Could you check a few things on this drawing? It's one solid part, dimensions in mm from its lowest x, y, z. A direction names the side the tool comes from. Round coordinates to 2 decimals unless told otherwise and drop trailing zeros. Write each loop counter-clockwise with the first axis right and the second up, starting at its lowest first coordinate (ties: lowest second). Pieces come first, ordered by that corner, then holes. Notation, with made-up numbers: (-27.5, 62) - (28.5, 62) arc R20 ccw to (28.5, 84) - close; hole circle Ø11 at (-6.5, 19.5). An arc over 180 degrees is marked (long way). Write item = value, one per line. Start each with the question number.
Item 1: If we section it at D-D (z = 48): Please give me the cut outline in (x, y), and give its area (3 significant figures).
Item 2: For P1, Ø24, axis at x = 50, z = 32, coming from the +Y side; P2, Ø5, axis at y = 9.5, z = 37.5, coming from the -X side; P3, Ø4, axis at x = 17, y = 3.5, coming from the -Z side; P4, Ø1.5, axis at x = 9.5, y = 8, coming from the +Z side, each with a flat end and sliding along its axis, tell me the tip position at first contact or that it passes through.
Item 3: If we section it at A-A (y = 12): Please give me the cut outline in (x, z).
Item 4: Thinking about a two-plate mould opening in Z: for the marked faces 5, 6 and 7, which applies, pulls with the +Z half, pulls with the -Z half, needs draft (parallel to the pull), parting line crosses it, or undercut?
Item 5: If I drill on line 1 along Z through (x, y) = (68, 18.8); line 2 along Z through (x, y) = (58, 3.05); line 3 along X through (y, z) = (19, 48.5), over which ranges is the centre line in solid material (lowest first)? Write a range as [from, to].
Item 6: Which directions (+Z, -Z, +X, -X, +Y, -Y) give clear straight access to the entire face, cutting with the end or side of a thin tool? Please do the marked faces 1, 2, 3 and 4.
Item 7: If we section it at C-C (z = 16): Please give me the cut outline in (x, y).
Item 8: If we section it at B-B (x = 58): Please give me the cut outline in (y, z), and give its area (3 significant figures).
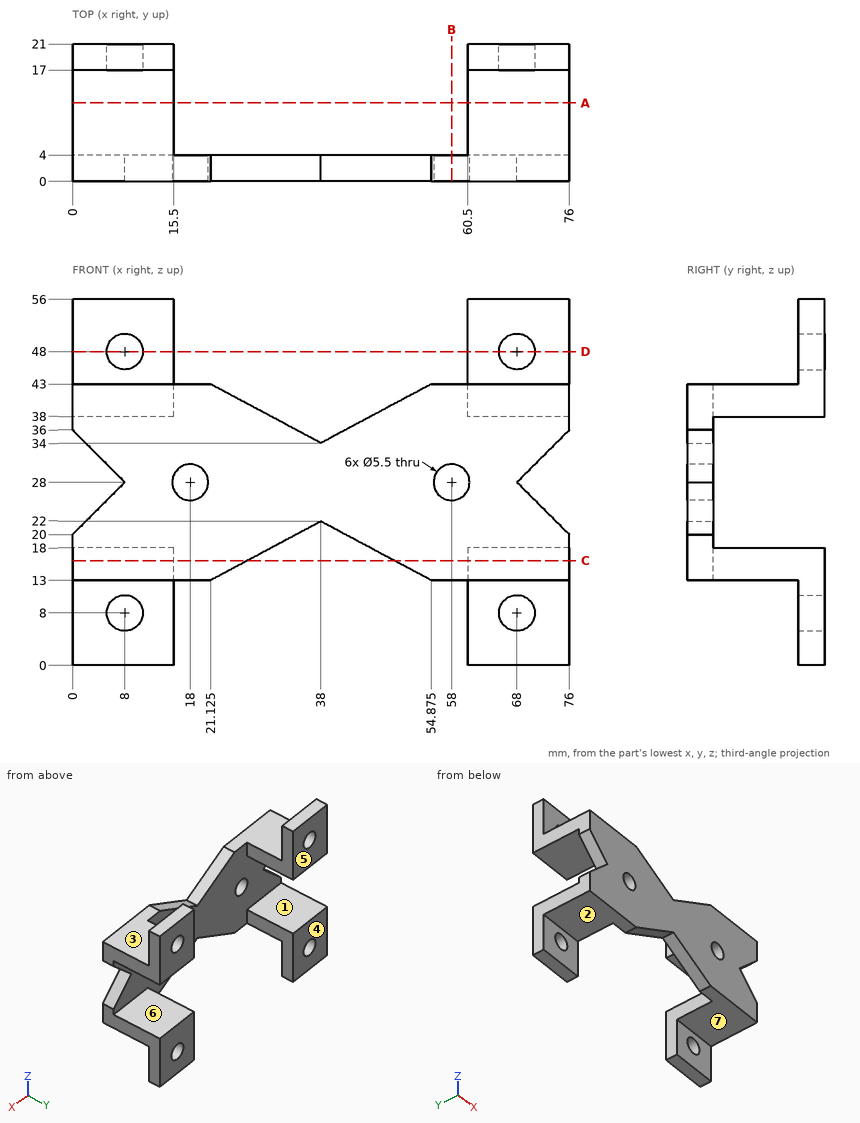
Reply:
q1.outline = (0, 17) - (5.25, 17) - (5.25, 21) - (0, 21) - close; (10.75, 17) - (15.5, 17) - (15.5, 21) - (10.75, 21) - close; (60.5, 17) - (65.25, 17) - (65.25, 21) - (60.5, 21) - close; (70.75, 17) - (76, 17) - (76, 21) - (70.75, 21) - close
q1.area = 80.0 mm2
q2.P1 = 4
q2.P2 = 0
q2.P3 = 13
q2.P4 = 43
q3.outline = (0, 13) - (15.5, 13) - (15.5, 18) - (0, 18) - close; (0, 38) - (15.5, 38) - (15.5, 43) - (0, 43) - close; (60.5, 13) - (76, 13) - (76, 18) - (60.5, 18) - close; (60.5, 38) - (76, 38) - (76, 43) - (60.5, 43) - close
q4.face_5 = needs draft
q4.face_6 = undercut
q4.face_7 = pulls with the -Z half
q5.line_1 = [0, 5.25], [10.75, 18], [38, 45.25], [50.75, 56]
q5.line_2 = [13, 25.25], [30.75, 43]
q5.line_3 = [0, 5.3], [10.7, 15.5], [60.5, 65.3], [70.7, 76]
q6.face_1 = +X, -X, +Y
q6.face_2 = -Z, +X, -X, -Y
q6.face_3 = +Z, +X, -X, -Y
q6.face_4 = +Z, -Z, +X, -X, +Y
q7.outline = (0, 0) - (26.75, 0) - (26.75, 4) - (15.5, 4) - (15.5, 21) - (0, 21) - close; (49.25, 0) - (76, 0) - (76, 21) - (60.5, 21) - (60.5, 4) - (49.25, 4) - close
q8.outline = (0, 13) - (4, 13) - (4, 25.25) - (0, 25.25) - close; (0, 30.75) - (4, 30.75) - (4, 43) - (0, 43) - close
q8.area = 98.0 mm2
